Job drawing, mm, ordinate dimensions from the low corner. One solid piece. Round coordinates to 2 decimals unless told otherwise and drop trailing zeros. Loops run counter-clockwise (first coordinate to the right, second up) from the corner with the lowest first, then second, coordinate; pieces in that order, holes last.
1) Probe line 1 (Y direction, x = 77, z = 1.7); line 2 (Y direction, x = 79, z = 2.85) (1 decimal); line 3 (X direction, y = 3, z = 0.3) (1 decimal). List the from-to ranges inside material, lowest first.
2) Drop a flat-ended pin along its axis: P1, Ø3, axis at x = 77, y = 32, coming from the +Z side. Give the stop position or say it passes through.
3) Band-saw the part on B-B, the plane y = 23. Write the cut outline in (x, z).
4) Band-saw the part on C-C, the plane x = 22. Write the cut outline in (y, z).
5) Band-saw the part on D-D, the plane y = 14. Write the cut outline in (x, z), then the cut area to 3 significant figures.
6) Band-saw the part on A-A, the plane z = 2.5. Write the cut outline in (x, y).
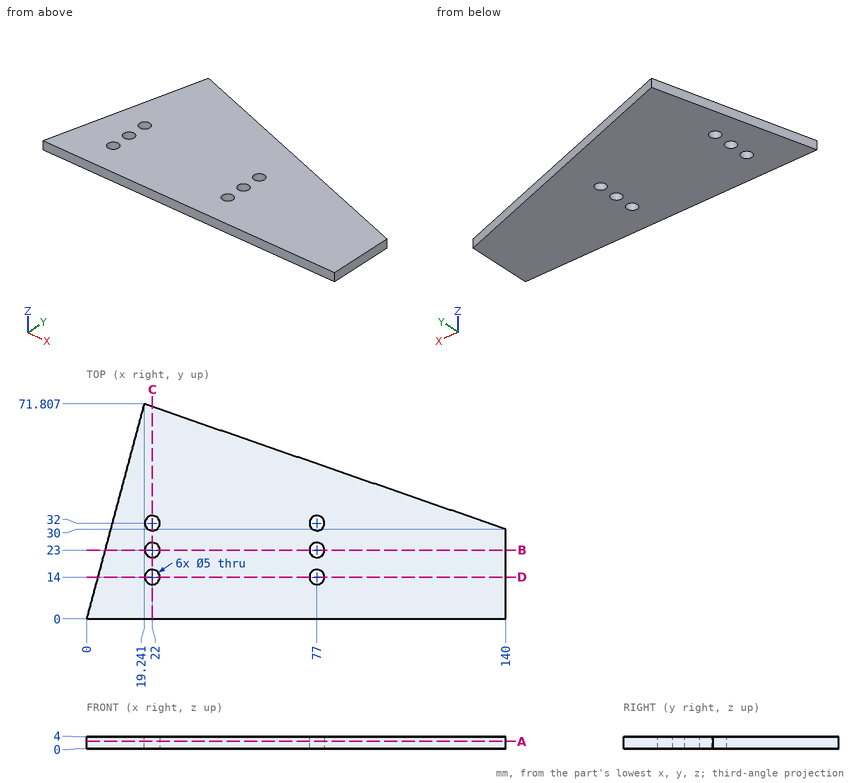
Reported:
1. line 1: y = 0 to 11.5, 16.5 to 20.5, 25.5 to 29.5, 34.5 to 51.81
1. line 2: y = 0 to 12.5, 15.5 to 21.5, 24.5 to 30.5, 33.5 to 51.1
1. line 3: x = 0.8 to 140
2. P1: passes through
3. outline: (6.16, 0) - (19.5, 0) - (19.5, 4) - (6.16, 4) - close; (24.5, 0) - (74.5, 0) - (74.5, 4) - (24.5, 4) - close; (79.5, 0) - (140, 0) - (140, 4) - (79.5, 4) - close
4. outline: (0, 0) - (11.5, 0) - (11.5, 4) - (0, 4) - close; (16.5, 0) - (20.5, 0) - (20.5, 4) - (16.5, 4) - close; (25.5, 0) - (29.5, 0) - (29.5, 4) - (25.5, 4) - close; (34.5, 0) - (70.85, 0) - (70.85, 4) - (34.5, 4) - close
5. outline: (3.75, 0) - (19.5, 0) - (19.5, 4) - (3.75, 4) - close; (24.5, 0) - (74.5, 0) - (74.5, 4) - (24.5, 4) - close; (79.5, 0) - (140, 0) - (140, 4) - (79.5, 4) - close
5. area: 505 mm2
6. outline: (0, 0) - (140, 0) - (140, 30) - (19.24, 71.81) - close; hole circle Ø5 at (22, 14); hole circle Ø5 at (22, 23); hole circle Ø5 at (22, 32); hole circle Ø5 at (77, 14); hole circle Ø5 at (77, 23); hole circle Ø5 at (77, 32)
